```python
from build123d import *

# Parameters (mm, degrees)
SKETCH1_R           = 25.4
BOSS_EXTRUDE1_DEPTH = 6.35
SKETCH2_R           = 1.5875
BOSS_EXTRUDE2_DEPTH = 12.7
CIRPATTERN1_COUNT   = 4
SKETCH3_R           = 3.175
CUT_EXTRUDE1_DEPTH  = 41.659838908
CIRPATTERN2_COUNT   = 4


with BuildPart() as part:
    # Sketch1 → Boss-Extrude1 (new body)
    with BuildSketch(Plane(origin=(0, 0, 0), x_dir=(1, 0, 0), z_dir=(0, 1, 0))):
        with Locations(Location((0, 0, 0), (0, 0, 270))):
            Circle(SKETCH1_R)
    extrude(amount=BOSS_EXTRUDE1_DEPTH)

    # Sketch2 → Boss-Extrude2 (add)
    with BuildSketch(Plane(origin=(0, 6.35, 0), x_dir=(1, 0, 0), z_dir=(0, 1, 0))):
        with Locations(Location((-19.05, 0, 0), (0, 0, 270))):
            Circle(SKETCH2_R)
    boss_extrude2 = extrude(amount=BOSS_EXTRUDE2_DEPTH)

    # CirPattern1: Boss-Extrude2 ×4 about axis
    cirpattern1_axis = Axis((0, 0, 0), (0, 1, 0))
    for i in range(1, CIRPATTERN1_COUNT):
        add(boss_extrude2.rotate(cirpattern1_axis, i * 360 / CIRPATTERN1_COUNT))

    # Sketch3 → Cut-Extrude1 (cut, through all)
    with BuildSketch(Plane.XZ):
        with Locations(Location((8.980256121, -8.980256121, 0), (0, 0, 270))):
            Circle(SKETCH3_R)
    cut_extrude1 = extrude(amount=-CUT_EXTRUDE1_DEPTH, mode=Mode.SUBTRACT)

    # CirPattern2: Cut-Extrude1 ×4 about axis
    cirpattern2_axis = Axis((0, 0, 0), (0, 1, 0))
    for i in range(1, CIRPATTERN2_COUNT):
        add(cut_extrude1.rotate(cirpattern2_axis, i * 360 / CIRPATTERN2_COUNT), mode=Mode.SUBTRACT)


solid = part.part
```
Verification items for the finished model (mm, model axes). A direction names the side the tool comes from. Coordinates: 2 decimals unless noted, no trailing zeros. Write each loop counter-clockwise with the first axis right and the second up, starting at its lowest first coordinate (ties: lowest second). Pieces come first, ordered by that corner, then holes. Notation, with made-up numbers: M -37.75,-24 L -19.75,-24 A6 cw -19.75,-18 Z; hole C 28.25,17 d3. An arc over 180 degrees is marked long. One line per item, written item: value.
Item 1: Scan lines: line 1 along Z through (x, y) = (-8, 1.75); line 2 along Y through (x, z) = (-3, -3.5); line 3 along Z through (x, y) = (-9, 3.5). Record each from-to range of solid material in increasing order.
Check sheet entries:
line 1: z = -24.11 to -12, -5.96 to 5.96, 12 to 24.11
line 2: y = 0 to 6.35
line 3: z = -23.75 to -12.16, -5.81 to 5.81, 12.16 to 23.75
Item 2: Access from +Z, -Z, +X, -X, +Y, -Y to the whole of each face (thin tool, end or side, straight path). Record for faces 1 (the flat face through (0, 0, 0)), 2 (the cylindrical face through (0.85, 12.61, 17.71)).
Check sheet entries:
face 1: +Z, -Z, +X, -X, -Y
face 2: +Y
Item 3: Section check B-B, the plane z = 0. Record the boundary of the cut face in (x, y), plus the area to 3 significant figures.
Check sheet entries:
outline: M -25.4,0 L 25.4,0 L 25.4,6.35 L 20.64,6.35 L 20.64,19.05 L 17.46,19.05 L 17.46,6.35 L -17.46,6.35 L -17.46,19.05 L -20.64,19.05 L -20.64,6.35 L -25.4,6.35 Z
area: 403 mm^2
Item 4: Section check D-D, the plane y = 3.5. Record the boundary of the cut face in (x, z) (3 decimals).
Check sheet entries:
outline: C 0,0 d50.8; hole C -8.98,-8.98 d6.35; hole C -8.98,8.98 d6.35; hole C 8.98,-8.98 d6.35; hole C 8.98,8.98 d6.35
Item 5: Gauge pin test, flat ends, axial feed: pin 1 Ø5.5 at (x, z) = (8.98, 8.98) entering from +Y; pin 2 Ø5 at (x, y) = (17, 7) entering from -Z; pin 3 Ø5 at (x, y) = (17.5, 7) entering from +Z; pin 4 Ø6 at (y, z) = (6, 17) entering from -X. Record the tip position at first contact, or that the pin passes through.
Check sheet entries:
pin 1: passes through
pin 2: stops at z = -20.79
pin 3: stops at z = 20.43
pin 4: stops at x = -21.19
Item 6: Section check A-A, the plane x = 0. Record the boundary of the cut face in (y, z), plus the area to 3 significant figures.
Check sheet entries:
outline: M 0,-25.4 L 6.35,-25.4 L 6.35,-20.64 L 19.05,-20.64 L 19.05,-17.46 L 6.35,-17.46 L 6.35,17.46 L 19.05,17.46 L 19.05,20.64 L 6.35,20.64 L 6.35,25.4 L 0,25.4 Z
area: 403 mm^2
Item 7: Section check C-C, the plane y = 15.5. State how many separate pieces and enclosed holes the cut face has, plus the area to 3 significant figures.
Check sheet entries:
separate pieces: 4
enclosed holes: 0
area: 31.7 mm^2
Item 8: Mould release check, pull along X, two halves, no side actions. Record for faces 3 (the cylindrical face through (-15.456, 3.131, -20.157)), 4 (the flat face through (19, 19.05, 0)), 5 (the cylindrical face through (17.71, 12.61, -0.85)): pulls with the +X half, pulls with the -X half, needs draft (parallel to the pull), parting line crosses it, or undercut.
Check sheet entries:
face 3: parting line crosses it
face 4: needs draft
face 5: undercut
